from build123d import *

# Parameters (mm, degrees)
F0_W     = 100
F0_H     = 20
F1_DEPTH = 120
F2_R     = 3
F3_DEPTH = 12
F4_R     = 3
F5_DEPTH = 12


with BuildPart() as f1:
    # F0 (on Top) → F1 (new body)
    with BuildSketch(Plane.XY):
        with Locations((50, 10)):
            Rectangle(F0_W, F0_H)
    extrude(amount=F1_DEPTH)

    # F2 (on face) → F3 (cut)
    with BuildSketch(Plane(origin=(0, 20, 0), x_dir=(-1, 0, 0), z_dir=(0, 1, 0))):
        with Locations((-50, 110)):
            Circle(F2_R)
    extrude(amount=-F3_DEPTH, mode=Mode.SUBTRACT)

    # F4 (on face) → F5 (cut)
    with BuildSketch(Plane(origin=(0, 20, 0), x_dir=(-1, 0, 0), z_dir=(0, 1, 0))):
        with Locations((-50, 10)):
            Circle(F4_R)
    extrude(amount=-F5_DEPTH, mode=Mode.SUBTRACT)


solid = f1.part
CAD build for the part. Positions are in the model's coordinates, mm. A direction names the side the tool comes from. Give positions to 0.01 mm unless a question says otherwise; leave off trailing zeros. Order: outer loops, then holes, each group sorted by start corner. A loop starts at its lowest first (then second) coordinate and runs counter-clockwise, first axis right, second up. Notation, with made-up numbers: (65, 78) - (109, 78) arc R25 ccw to (109, 113) - close; hole circle Ø8 at (80.25, 76). An arc over 180 degrees is marked (long way). Answer in a Markdown table with one row per item.
1. Probe probe 1 along Z at (x, y) = (50, 13.75). List the from-to ranges inside material, lowest first. Write a range as [from, to].
Data:
| item | result |
|---|---|
| probe 1 | z = [0, 7], [13, 107], [113, 120] |
2. Flat gauge pin, fed straight in: pin 1 (5.5 mm diameter, centred on x = 50, z = 110, fed in from +Y). Where does the tip first touch, or does it go through?
Data:
| item | result |
|---|---|
| pin 1 | stops at y = 8 |
3. Pull direction X, two halves, no side cores. Call faces 3 (the flat face through (100, 10, 59)), 4 (the flat face through (49, 10, 120)), 5 (the cylindrical face through (53, 14, 110)): pulls with the +X half, pulls with the -X half, needs draft (parallel to the pull), parting line crosses it, or undercut.
Data:
| item | result |
|---|---|
| face 3 | pulls with the +X half |
| face 4 | needs draft |
| face 5 | undercut |
4. Tool access for faces 1 (the flat face through (0, 10, 59)), 2 (the flat face through (50, 8, 10)): list every direction of +Z, -Z, +X, -X, +Y, -Y with a clear straight run to the whole face (end or side of a thin tool).
Data:
| item | result |
|---|---|
| face 1 | +Z, -Z, -X, +Y, -Y |
| face 2 | +Y |
5. Saw through at B-B, the plane x = 50. Give the cut face in (y, z).
Data:
| item | result |
|---|---|
| outline | (0, 0) - (20, 0) - (20, 7) - (8, 7) - (8, 13) - (20, 13) - (20, 107) - (8, 107) - (8, 113) - (20, 113) - (20, 120) - (0, 120) - close |
6. Saw through at A-A, the plane z = 10. Give the cut face in (x, y).
Data:
| item | result |
|---|---|
| outline | (0, 0) - (100, 0) - (100, 20) - (53, 20) - (53, 8) - (47, 8) - (47, 20) - (0, 20) - close |
